from build123d import *

# Parameters (mm, degrees)
F0_W     = 57.15
F0_H     = 76.2
F1_DEPTH = 38.1
F2_T     = -2.54
F3_W     = 15.24
F3_H     = 11.43
F4_DEPTH = 25.4
F6_D     = 8.128
F6_DEPTH = 12.7


with BuildPart() as f1:
    # F0 (on Top) → F1 (new body)
    with BuildSketch(Plane.XY):
        Rectangle(F0_W, F0_H)
    extrude(amount=F1_DEPTH)

    # F2
    f2_openings = [f1.faces().sort_by_distance(p)[0] for p in [
        (0, 0, 38.1),
    ]]
    offset(amount=F2_T, openings=f2_openings)

    # F3 (on face) → F4 (cut)
    with BuildSketch(Plane.YZ.offset(28.575)):
        with Locations((-18.261918, 24.186697)):
            Rectangle(F3_W, F3_H)
    extrude(amount=-F4_DEPTH, mode=Mode.SUBTRACT)

    # F6
    with Locations(Plane.YZ.offset(28.575)):
        with Locations((17.349107, 24.799019)):
            Hole(F6_D / 2, depth=F6_DEPTH)


solid = f1.part
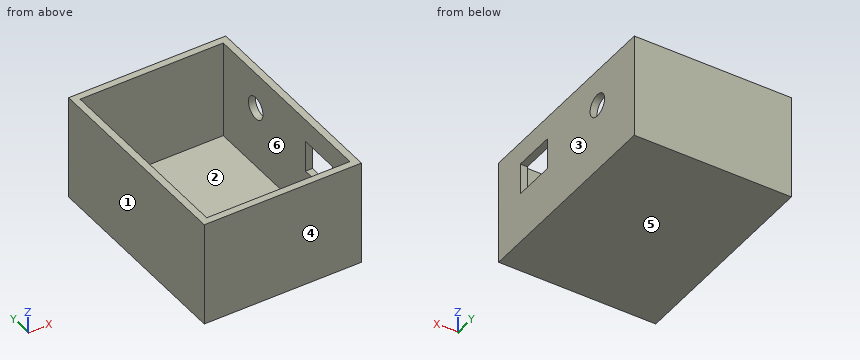
Can you work these out from the model? Positions are in its coordinate system, mm. Face numbers are marked on the shaded views. A direction names the side the tool comes from. Coordinates: 2 decimals unless noted, no trailing zeros. Write each loop counter-clockwise with the first axis right and the second up, starting at its lowest first coordinate (ties: lowest second). Pieces come first, ordered by that corner, then holes.
Q1. Imagine slicing it at A-A, the plane z = 26. List the corners of the cut face in (x, y) for me (3 decimals), plus the area to 3 significant figures.
Results found:
outline: (-28.575, -38.1) - (28.575, -38.1) - (28.575, -25.882) - (26.035, -25.882) - (26.035, -35.56) - (-26.035, -35.56) - (-26.035, 35.56) - (26.035, 35.56) - (26.035, 21.232) - (28.575, 21.232) - (28.575, 38.1) - (-28.575, 38.1) - close; (26.035, -10.642) - (28.575, -10.642) - (28.575, 13.467) - (26.035, 13.467) - close
area: 593 mm2
Q2. Imagine slicing it at C-C, the plane z = 13.5. List the corners of the cut face in (x, y) for me (3 decimals).
Results found:
outline: (-28.575, -38.1) - (28.575, -38.1) - (28.575, 38.1) - (-28.575, 38.1) - close; hole (-26.035, -35.56) - (26.035, -35.56) - (26.035, 35.56) - (-26.035, 35.56) - close
Q3. Imagine slicing it at B-B, the plane y = 14.5. List the corners of the cut face in (x, z) for me (3 decimals).
Results found:
outline: (-28.575, 0) - (28.575, 0) - (28.575, 21.901) - (26.035, 21.901) - (26.035, 2.54) - (-26.035, 2.54) - (-26.035, 38.1) - (-28.575, 38.1) - close; (26.035, 27.697) - (28.575, 27.697) - (28.575, 38.1) - (26.035, 38.1) - close
Q4. For P1, Ø0.8, axis at x = 28, y = -17.5, coming from the -Z side; P2, Ø4, axis at x = -8.5, y = 27.5, coming from the +Z side, each with a flat end and sliding along its axis, tell me the tip position at first contact or that it passes through.
Results found:
P1: stops at z = 0
P2: stops at z = 2.54
Q5. Imagine slicing it at D-D, the plane x = 17. List the corners of the cut face in (y, z) for me.
Results found:
outline: (-38.1, 0) - (38.1, 0) - (38.1, 38.1) - (35.56, 38.1) - (35.56, 2.54) - (-35.56, 2.54) - (-35.56, 38.1) - (-38.1, 38.1) - close
Q6. If we mould it in two halves opening along X, with no side actions, what happens to the marked faces 1, 2, 3 and 4? For each: +X half, -X half, draft (parallel to the pull), parting line (faces both ways), or undercut.
Results found:
face 1: -X half
face 2: undercut
face 3: +X half
face 4: draft
Q7. Please list where these lines run through material, in increasing order: L1, parallel to Y at x = -22.5, z = 18; L2, parallel to X at y = 15.5, z = 14 (3 decimals); L3, parallel to X at y = 16, z = 25.5 (3 decimals).
Results found:
L1: y = -38.1 to -35.56, 35.56 to 38.1
L2: x = -28.575 to -26.035, 26.035 to 28.575
L3: x = -28.575 to -26.035
Q8. Which directions (+Z, -Z, +X, -X, +Y, -Y) give clear straight access to the entire face, cutting with the end or side of a thin tool? Please do the marked faces 5 and 6.
Results found:
face 5: -Z, +X, -X, +Y, -Y
face 6: +Z
